Verification items for the finished model (mm, model axes). A direction names the side the tool comes from. Give positions to 0.01 mm unless a question says otherwise; leave off trailing zeros. Order: outer loops, then holes, each group sorted by start corner. A loop starts at its lowest first (then second) coordinate and runs counter-clockwise, first axis right, second up.
(1) Sectioned sample at A-A on x = 8.75. Record the cut outline in (y, z), plus the area to 3 significant figures.
(2) Mould release check, pull along X, two halves, no side actions. Record for faces 3 (the face through (14, 0, 2)), 4 (the face through (28, 13, 2)), 5 (the face through (3.15, 5.44, 0.49)): pulls with the +X half, pulls with the -X half, needs draft (parallel to the pull), parting line crosses it, or undercut.
(3) Access from +Z, -Z, +X, -X, +Y, -Y to the whole of each face (thin tool, end or side, straight path). Record for faces 1 (the face through (24.15, 5.44, 0.49)), 2 (the face through (5, 17, 1)).
(4) Scan lines: L1, parallel to Y at x = 24.5, z = 1.85; L2, parallel to Y at x = 24.5, z = 0.3; L3, parallel to X at y = 19.5, z = 1.05. Record each from-to range of solid material in increasing order.
(5) Sectioned sample at C-C on y = 18.4. Record the cut outline in (x, z).
(6) Gauge pin test, flat ends, axial feed: pin 1 (4 mm diameter, centred on x = 24.5, y = 7, fed in from +Z); pin 2 (3 mm diameter, centred on x = 3.5, y = 7, fed in from +Z). Record the tip position at first contact, or that the pin passes through.
(7) Sectioned sample at B-B on z = 2.75. Count the separate pieces of the cut face and the enclosed holes in it, plus the area to 3 significant figures.
```python
from build123d import *

# Parameters (mm, degrees)
SKETCH1_W           = 28
SKETCH1_H           = 25.4
SKETCH1_R           = 1.25
SKETCH1_R_2         = 1.6
BOSS_EXTRUDE1_DEPTH = 4
SKETCH2_R           = 3
CUT_EXTRUDE1_DEPTH  = 3


with BuildPart() as part:
    # Sketch1 → Boss-Extrude1 (new body)
    with BuildSketch(Plane.XY):
        with Locations((14, 12.7)):
            Rectangle(SKETCH1_W, SKETCH1_H)
        with Locations((8.75, 17.95)):
            Circle(SKETCH1_R, mode=Mode.SUBTRACT)
        with Locations((19.25, 17.95)):
            Circle(SKETCH1_R, mode=Mode.SUBTRACT)
        with Locations((19.25, 7.45)):
            Circle(SKETCH1_R, mode=Mode.SUBTRACT)
        with Locations((8.75, 7.45)):
            Circle(SKETCH1_R, mode=Mode.SUBTRACT)
        with Locations((3.5, 18.4)):
            Circle(SKETCH1_R_2, mode=Mode.SUBTRACT)
        with Locations((3.5, 7)):
            Circle(SKETCH1_R_2, mode=Mode.SUBTRACT)
        with Locations((24.5, 7)):
            Circle(SKETCH1_R_2, mode=Mode.SUBTRACT)
        with Locations((24.5, 18.4)):
            Circle(SKETCH1_R_2, mode=Mode.SUBTRACT)
    extrude(amount=BOSS_EXTRUDE1_DEPTH)

    # Sketch2 → Cut-Extrude1 (cut)
    with BuildSketch(Plane.XY.offset(4)):
        with Locations((24.5, 18.4)):
            Circle(SKETCH2_R)
        with Locations((3.5, 18.4)):
            Circle(SKETCH2_R)
        with Locations((3.5, 7)):
            Circle(SKETCH2_R)
        with Locations((24.5, 7)):
            Circle(SKETCH2_R)
    extrude(amount=-CUT_EXTRUDE1_DEPTH, mode=Mode.SUBTRACT)


solid = part.part
```
Ans:
1. outline: (0, 0) - (6.2, 0) - (6.2, 4) - (0, 4) - close; (8.7, 0) - (16.7, 0) - (16.7, 4) - (8.7, 4) - close; (19.2, 0) - (25.4, 0) - (25.4, 4) - (19.2, 4) - close
1. area: 81.6 mm2
2. face 3: needs draft
2. face 4: pulls with the +X half
2. face 5: undercut
3. face 1: +Z, -Z
3. face 2: +Z
4. L1: y = 0 to 4, 10 to 15.4, 21.4 to 25.4
4. L2: y = 0 to 5.4, 8.6 to 16.8, 20 to 25.4
4. L3: x = 0 to 0.71, 6.29 to 21.71, 27.29 to 28
5. outline: (0, 0) - (1.9, 0) - (1.9, 1) - (0.5, 1) - (0.5, 4) - (0, 4) - close; (5.1, 0) - (7.58, 0) - (7.58, 4) - (6.5, 4) - (6.5, 1) - (5.1, 1) - close; (9.92, 0) - (18.08, 0) - (18.08, 4) - (9.92, 4) - close; (20.42, 0) - (22.9, 0) - (22.9, 1) - (21.5, 1) - (21.5, 4) - (20.42, 4) - close; (26.1, 0) - (28, 0) - (28, 4) - (27.5, 4) - (27.5, 1) - (26.1, 1) - close
6. pin 1: stops at z = 1
6. pin 2: passes through
7. separate pieces: 1
7. enclosed holes: 8
7. area: 578 mm2
